Autodesk Inventor part; units mm, degrees
ref_plane "YZ Plane" through (0, 0, 0) normal (1, 0, 0) x (0, 1, 0)
ref_plane "XZ Plane" through (0, 0, 0) normal (0, 1, 0) x (-1, 0, 0)
ref_plane "XY Plane" through (0, 0, 0) normal (0, 0, 1) x (1, 0, 0)
sketch "スケッチ7" plane through (0, 0, 0) normal (0, 1, 0) x (-1, 0, 0)
  circle A0 centre (0, 0) radius 25
  dimension "d28" = 50
extrude "押し出し4" add sketch "スケッチ7" along normal blind 44.5
sketch "スケッチ8" plane through (0, 44.5, 0) normal (0, 1, 0) x (1, 0, 0)
  circle A0 centre (0, 0) radius 4
  dimension "d31" = 8
extrude "押し出し5" add sketch "スケッチ8" along normal blind 36.7
sketch "スケッチ9" plane through (0, 0, 0) normal (0, -1, 0) x (1, 0, 0)
  line L0 (0, 0) -> (7.0711, -7.0711)
  line L1 (0, 0) -> (10, 0) construction
  point P0 (7.0711, 7.0711)
  point P1 (-7.0711, 7.0711)
  point P2 (-7.0711, -7.0711)
  dimension "d34" = 10
  dimension "d35" = 45
  dimension "d38" = 360
hole "穴2" at (7.0711, 0, -7.0711) at (7.0711, 0, 7.0711) at (-7.0711, 0, 7.0711) at (-7.0711, 0, -7.0711) direction (0, 1, 0) diameter 2.459 depth 8.8 tip angle 118
sketch "スケッチ11" plane through (0, 0, 0) normal (0, -1, 0) x (1, 0, 0)
  circle A0 centre (0, 0) radius 7
  dimension "d52" = 14
extrude "押し出し7" add sketch "スケッチ11" along normal blind 2
properties part number "Rotar" material "アルミニウム 6061"
Read the model definition and answer for the solid it produces. Units are mm, in the model's axes. A direction names the side the tool comes from. Coordinates: 2 decimals unless noted, no trailing zeros. Order: outer loops, then holes, each group sorted by start corner. A loop starts at its lowest first (then second) coordinate and runs counter-clockwise, first axis right, second up. Notation, with made-up numbers: M -19,-10 L 24,-10 A17 cw 24,22 Z; hole C 28,45 d2. An arc over 180 degrees is marked long. Put each result on its own line as item: value. Start each with the question number.
Item 1: Consider probe 1 along Y at (x, z) = (4.5, 22.5); probe 2 along Y at (x, z) = (3, 4.5); probe 3 along X at (y, z) = (14.5, -0.5) (3 decimals). Determine where each line is inside the solid, lowest interval first. Write a range as [from, to].
Item 2: Section B-B, the plane z = 0 is taken. Determine the outline of the cut face in (x, y).
Item 3: Section C-C, the plane y = 4 is taken. Determine the outline of the cut face in (x, z).
Item 4: Section D-D, the plane y = 32 is taken. Determine the outline of the cut face in (x, z), plus the area to 3 significant figures.
Item 5: Section A-A, the plane x = 0 is taken. Determine the outline of the cut face in (y, z).
Item 6: For faces 1 (the face through (-0.867, 62.593, -3.905)), 2 (the face through (0, -2, 0)), 3 (the face through (8.16, 4.46, 6.5)), determine the directions among +Z, -Z, +X, -X, +Y, -Y from which every point of the face is accessible in a straight line to the end or side of a thin tool.
Item 7: Given pin 1 Ø10 at (y, z) = (48.5, 5) entering from +X; pin 2 Ø12 at (x, y) = (6.5, 7) entering from +Z (3 decimals); pin 3 Ø4 at (x, z) = (-7.07, 7.07) entering from +Y, each flat-ended and moving along its own axis, determine where each tip first touches the part or whether it passes through.
Item 8: The mould has two halves that part along X. Classify faces 4 (the face through (6.466, -0.986, 2.681)), 5 (the face through (6.88, 9.41, 6.97)), 6 (the face through (0, 44.5, -5)): +X half, -X half, draft (parallel to the pull), parting line (faces both ways), or undercut.
Computed:
1. probe 1: y = [0, 44.5]
1. probe 2: y = [-2, 44.5]
1. probe 3: x = [-24.995, 24.995]
2. outline: M -25,0 L -7,0 L -7,-2 L 7,-2 L 7,0 L 25,0 L 25,44.5 L 4,44.5 L 4,81.2 L -4,81.2 L -4,44.5 L -25,44.5 Z
3. outline: C 0,0 d50; hole C -7.07,-7.07 d2.46; hole C -7.07,7.07 d2.46; hole C 7.07,-7.07 d2.46; hole C 7.07,7.07 d2.46
4. outline: C 0,0 d50
4. area: 1,960 mm2
5. outline: M -2,-7 L 0,-7 L 0,-25 L 44.5,-25 L 44.5,-4 L 81.2,-4 L 81.2,4 L 44.5,4 L 44.5,25 L 0,25 L 0,7 L -2,7 Z
6. face 1: +Y
6. face 2: +Z, -Z, +X, -X, -Y
6. face 3: -Y
7. pin 1: stops at x = 24.92
7. pin 2: stops at z = 24.995
7. pin 3: stops at y = 44.5
8. face 4: parting line
8. face 5: undercut
8. face 6: draft
